For this review, take the finished solid that the model builds, in its own axes (mm). A direction names the side the tool comes from. Round coordinates to 2 decimals unless told otherwise and drop trailing zeros. Write each loop counter-clockwise with the first axis right and the second up, starting at its lowest first coordinate (ties: lowest second). Pieces come first, ordered by that corner, then holes. Notation, with made-up numbers: (-18, 36.5) - (-13, 36.5) arc R21 cw to (-13, 74.5) - close; hole circle Ø7 at (49, 31.5). An arc over 180 degrees is marked (long way). Answer in a Markdown table with one row per item. Add a question column.
from build123d import *

# Parameters (mm, degrees)
BOSS_EXTRUDE1_DEPTH             = 20
SKETCH6_R                       = 12.25
BOSS_EXTRUDE2_DEPTH             = 4.5
SKETCH4_W                       = 157.727290237
SKETCH4_H                       = 50
CUT_EXTRUDE10_DEPTH             = 34.640665044
CUT_EXTRUDE12_DEPTH             = 141.625104537
CUT_EXTRUDE12_DEPTH_BACK        = 141.625104537
SKETCH11_R                      = 10.625
SKETCH11_R_2                    = 0.95
SKETCH11_R_3                    = 0.675
CUT_EXTRUDE13_DEPTH             = 2
SKETCH12_R                      = 3.5
SKETCH12_R_2                    = 0.95
CUT_EXTRUDE14_DEPTH             = 1
CUT_EXTRUDE15_REACH             = 153.797
SKETCH14_R                      = 5
CUT_EXTRUDE16_DEPTH             = 124.889930448
CUT_EXTRUDE17_DEPTH             = 108.475579093
CUT_EXTRUDE17_DRAFT             = -2.1
CUT_EXTRUDE17_PROFILE_2_DEPTH   = 108.475579093
CUT_EXTRUDE17_PROFILE_2_DRAFT   = -2.1
CUT_EXTRUDE18_REACH             = 151.086
SKETCH16_R                      = 1
SKETCH18_R                      = 6.25
BOSS_EXTRUDE4_DEPTH             = 5.5
BOSS_EXTRUDE4_DEPTH_BACK        = 4
SKETCH19_W                      = 13
SKETCH19_H                      = 3.5
BOSS_EXTRUDE5_DEPTH             = 21.3
BOSS_EXTRUDE5_DIRECTION_2_REACH = 125.89
SKETCH20_R                      = 7.5
BOSS_EXTRUDE6_DEPTH             = 0.75
CUT_EXTRUDE19_REACH             = 153.797
SKETCH17_R                      = 3


with BuildPart() as part:
    # Sketch1 → Boss-Extrude1 (new, symmetric)
    with BuildSketch(Plane.YZ):
        Polygon((-14.772710004, -33), (35.227289996, -33), (135.227290242, -15.19542909), (135.227290242, -11.132523186), (105.227290242, -16.473894445), (105.227290242, 16.473894445), (135.227290242, 11.132523186), (135.227290242, 15.19542909), (35.227289996, 33), (-14.772710004, 33), (-14.772710004, 29), (34.917768753, 29), (34.917768753, -29), (-14.772710004, -29), align=None)
        Polygon((40.917768753, -27.923928772), (67.072529497, -23.267185861), (67.072529497, 23.267185861), (40.917768753, 27.923928772), align=None, mode=Mode.SUBTRACT)
        Polygon((73.072529497, 22.198911609), (99.227290242, 17.542168697), (99.227290242, -17.542168697), (73.072529497, -22.198911609), align=None, mode=Mode.SUBTRACT)
    extrude(amount=BOSS_EXTRUDE1_DEPTH, both=True)

    # Sketch6 → Boss-Extrude2 (add)
    with BuildSketch(Plane.XY.offset(-29)):
        Circle(SKETCH6_R)
    extrude(amount=BOSS_EXTRUDE2_DEPTH)

    # Sketch4 → Cut-Extrude10 (cut, symmetric)
    with BuildSketch(Plane(origin=(0, 0, 0), x_dir=(0, 1, 0), z_dir=(0, 0, 1))):
        with Locations((61.363645124, 0)):
            Rectangle(SKETCH4_W, SKETCH4_H)
        with BuildLine():
            Line((35.227289996, 20), (130.476978326, 15.237515595))
            ThreePointArc((130.476978326, 15.237515595), (133.850026805, 13.689879231), (135.227290242, 10.243753901))
            Line((135.227290242, 10.243753901), (135.227290242, -10.243753901))
            ThreePointArc((135.227290242, -10.243753901), (133.850026805, -13.689879231), (130.476978326, -15.237515595))
            Line((130.476978326, -15.237515595), (35.227289996, -20))
            Line((35.227289996, -20), (-2.499999995, -20))
            ThreePointArc((-2.499999995, -20), (-9.571067807, -17.071067812), (-12.499999995, -10))
            Line((-12.499999995, -10), (-12.499999995, 10))
            ThreePointArc((-12.499999995, 10), (-9.571067807, 17.071067812), (-2.499999995, 20))
            Line((-2.499999995, 20), (35.227289996, 20))
        make_face(mode=Mode.SUBTRACT)
    extrude(amount=CUT_EXTRUDE10_DEPTH, both=True, mode=Mode.SUBTRACT)

    # Sketch8 → Cut-Extrude12 (cut, two sides)
    with BuildSketch(Plane(origin=(0, 0, 0), x_dir=(0, 1, 0), z_dir=(0, 0, 1))) as cut_extrude12_sk:
        with BuildLine():
            Line((117.127290242, 4.875), (127.127290242, 4.875))
            ThreePointArc((127.127290242, 4.875), (132.002290242, 0), (127.127290242, -4.875))
            Line((127.127290242, -4.875), (117.127290242, -4.875))
            ThreePointArc((117.127290242, -4.875), (112.252290242, 0), (117.127290242, 4.875))
        make_face()
    extrude(amount=CUT_EXTRUDE12_DEPTH, mode=Mode.SUBTRACT)
    extrude(cut_extrude12_sk.sketch, amount=-CUT_EXTRUDE12_DEPTH_BACK, mode=Mode.SUBTRACT)

    # Sketch11 → Cut-Extrude13 (cut)
    with BuildSketch(Plane.XY.offset(-24.5)):
        Circle(SKETCH11_R)
        Circle(SKETCH11_R_2, mode=Mode.SUBTRACT)
        with Locations(Location((2.545584412, 7.353910524, 0), (0, 0, 180))):
            Circle(SKETCH11_R_3, mode=Mode.SUBTRACT)
        with Locations(Location((4.949747468, 4.949747468, 0), (0, 0, 180))):
            Circle(SKETCH11_R_3, mode=Mode.SUBTRACT)
        with Locations((-2.545584412, 7.353910524)):
            Circle(SKETCH11_R_3, mode=Mode.SUBTRACT)
        with Locations((-4.949747468, 4.949747468)):
            Circle(SKETCH11_R_3, mode=Mode.SUBTRACT)
        with Locations(Location((-7.353910524, 2.545584412, 0), (0, 0, 180))):
            Circle(SKETCH11_R_3, mode=Mode.SUBTRACT)
        with Locations(Location((-4.949747468, -4.949747468, 0), (0, 0, 180))):
            Circle(SKETCH11_R_3, mode=Mode.SUBTRACT)
        with Locations(Location((-2.545584412, -7.353910524, 0), (0, 0, 180))):
            Circle(SKETCH11_R_3, mode=Mode.SUBTRACT)
        with Locations(Location((7.353910524, -2.545584412, 0), (0, 0, 180))):
            Circle(SKETCH11_R_3, mode=Mode.SUBTRACT)
        with Locations((2.545584412, -7.353910524)):
            Circle(SKETCH11_R_3, mode=Mode.SUBTRACT)
        with Locations((4.949747468, -4.949747468)):
            Circle(SKETCH11_R_3, mode=Mode.SUBTRACT)
    extrude(amount=-CUT_EXTRUDE13_DEPTH, mode=Mode.SUBTRACT)

    # Sketch12 → Cut-Extrude14 (cut)
    with BuildSketch(Plane.XY.offset(-26.5)):
        Circle(SKETCH12_R)
        Circle(SKETCH12_R_2, mode=Mode.SUBTRACT)
    extrude(amount=-CUT_EXTRUDE14_DEPTH, mode=Mode.SUBTRACT)

    # Sketch13 → Cut-Extrude15 (cut, up to next)
    with BuildSketch(Plane(origin=(0, 0, -33), x_dir=(1, 0, 0), z_dir=(0, 0, -1)), mode=Mode.PRIVATE) as cut_extrude15_sk1:
        with BuildLine():
            Line((-9, 12.499999995), (-20, 12.499999995))
            Line((-20, 12.499999995), (-20, -21.500000005))
            ThreePointArc((-20, -21.500000005), (-19.160251472, -18.726499024), (-16.923076923, -16.88461539))
            ThreePointArc((-16.923076923, -16.88461539), (-13.343597645, -13.937601575), (-12, -9.500000005))
            Line((-12, -9.500000005), (-12, 9.499999995))
            ThreePointArc((-12, 9.499999995), (-11.121320344, 11.621320339), (-9, 12.499999995))
        make_face()
    cut_extrude15_tool1 = extrude(cut_extrude15_sk1.sketch, amount=-CUT_EXTRUDE15_REACH, mode=Mode.PRIVATE) & part.part
    add(cut_extrude15_tool1.solids().sort_by_distance((-16.130851, 1.777121, -33))[0], mode=Mode.SUBTRACT)

    # Sketch14 → Cut-Extrude16 (cut, through all)
    with BuildSketch(Plane(origin=(0, 105.227290242, 0), x_dir=(-1, 0, 0), z_dir=(0, 1, 0))):
        with Locations(Location((0, 0, 0), (0, 0, 90))):
            Circle(SKETCH14_R)
    extrude(amount=-CUT_EXTRUDE16_DEPTH, mode=Mode.SUBTRACT)


with BuildPart() as cut_extrude17_tool:
    # Sketch15 → Cut-Extrude17 (with draft: the straight prism first)
    with BuildSketch(Plane.XZ.offset(-34.917768753)):
        with BuildLine():
            Line((-22.502320086, 32.227030747), (-22.502320086, -32.227030747))
            ThreePointArc((-22.502320086, -32.227030747), (-10.730823709, 0), (-22.502320086, 32.227030747))
        make_face()
    extrude(amount=-CUT_EXTRUDE17_DEPTH)
    # Cut-Extrude17: the draft: its side faces are tilted about the plane it starts from
    cut_extrude17_sides = [cut_extrude17_tool.faces().sort_by_distance(p)[0] for p in [
        (-22.502320086, 89.155558299, 0),
        (-10.730823709, 89.155558299, 0),
    ]]
    draft(cut_extrude17_sides, Plane.XZ.offset(-34.917768753), CUT_EXTRUDE17_DRAFT)


with BuildPart() as part_1:
    add(part.part)

    # Cut-Extrude17: cut by cut_extrude17_tool
    add(cut_extrude17_tool.part, mode=Mode.SUBTRACT)


with BuildPart() as cut_extrude17_profile_2_tool:
    # Sketch15 → Cut-Extrude17 profile 2 (with draft: the straight prism first)
    with BuildSketch(Plane.XZ.offset(-34.917768753)):
        with BuildLine():
            ThreePointArc((22.502320086, 32.227030747), (10.730823709, 0), (22.502320086, -32.227030747))
            Line((22.502320086, -32.227030747), (22.502320086, 32.227030747))
        make_face()
    extrude(amount=-CUT_EXTRUDE17_PROFILE_2_DEPTH)
    # Cut-Extrude17 profile 2: the draft: its side faces are tilted about the plane it starts from
    cut_extrude17_profile_2_sides = [cut_extrude17_profile_2_tool.faces().sort_by_distance(p)[0] for p in [
        (22.502320086, 89.155558299, 0),
        (10.730823709, 89.155558299, 0),
    ]]
    draft(cut_extrude17_profile_2_sides, Plane.XZ.offset(-34.917768753), CUT_EXTRUDE17_PROFILE_2_DRAFT)


with BuildPart() as part_2:
    add(part_1.part)

    # Cut-Extrude17 profile 2: cut by cut_extrude17_profile_2_tool
    add(cut_extrude17_profile_2_tool.part, mode=Mode.SUBTRACT)

    # Sketch16 → Cut-Extrude18 (cut, up to next)
    with BuildSketch(Plane.XY.offset(-26.5), mode=Mode.PRIVATE) as cut_extrude18_sk1:
        with Locations((-7.353910524, -2.545584412)):
            Circle(SKETCH16_R)
    cut_extrude18_tool1 = extrude(cut_extrude18_sk1.sketch, amount=-CUT_EXTRUDE18_REACH, mode=Mode.PRIVATE) & part_2.part
    # Sketch16 → Cut-Extrude18 (cut, up to next)
    with BuildSketch(Plane.XY.offset(-26.5), mode=Mode.PRIVATE) as cut_extrude18_sk2:
        with Locations((7.353910524, 2.545584412)):
            Circle(SKETCH16_R)
    cut_extrude18_tool2 = extrude(cut_extrude18_sk2.sketch, amount=-CUT_EXTRUDE18_REACH, mode=Mode.PRIVATE) & part_2.part
    add(cut_extrude18_tool1.solids().sort_by_distance((-7.353911, -2.545584, -26.5))[0], mode=Mode.SUBTRACT)
    add(cut_extrude18_tool2.solids().sort_by_distance((7.353911, 2.545584, -26.5))[0], mode=Mode.SUBTRACT)

    # Sketch18 → Boss-Extrude4 (add, two sides)
    with BuildSketch(Plane(origin=(0, 0, 29), x_dir=(1, 0, 0), z_dir=(0, 0, -1))) as boss_extrude4_sk:
        with Locations(Location((0, 0, 0), (0, 0, 270))):
            Circle(SKETCH18_R)
    extrude(amount=BOSS_EXTRUDE4_DEPTH)
    extrude(boss_extrude4_sk.sketch, amount=-BOSS_EXTRUDE4_DEPTH_BACK)

    # Sketch19 → Boss-Extrude5 (add)
    with BuildSketch(Plane(origin=(0, 105.227290242, 0), x_dir=(-1, 0, 0), z_dir=(0, 1, 0))):
        Rectangle(SKETCH19_W, SKETCH19_H)
    extrude(amount=BOSS_EXTRUDE5_DEPTH)

    # Boss-Extrude5 direction 2: up to this face of the body (flat: up to its plane)
    boss_extrude5_direction_2_end = Plane(part_2.part.faces().sort_by_distance((0, 99.227290242, 17.061388609))[0])
    # Sketch19 → Boss-Extrude5 direction 2 (add, up to the picked face)
    with BuildSketch(Plane(origin=(0, 105.227290242, 0), x_dir=(-1, 0, 0), z_dir=(0, 1, 0)), mode=Mode.PRIVATE) as boss_extrude5_direction_2_sk1:
        Rectangle(SKETCH19_W, SKETCH19_H)
    boss_extrude5_direction_2_tool1 = split(extrude(boss_extrude5_direction_2_sk1.sketch, amount=-BOSS_EXTRUDE5_DIRECTION_2_REACH, mode=Mode.PRIVATE), bisect_by=boss_extrude5_direction_2_end, keep=Keep.BOTH, mode=Mode.PRIVATE)
    add(boss_extrude5_direction_2_tool1.solids().sort_by(Axis((0, 105.22729, 0), (0, -1, 0)))[0])

    # Sketch20 → Boss-Extrude6 (add)
    with BuildSketch(Plane(origin=(0, 0, 23.5), x_dir=(1, 0, 0), z_dir=(0, 0, -1))):
        with Locations(Location((0, 0, 0), (0, 0, 270))):
            Circle(SKETCH20_R)
    extrude(amount=-BOSS_EXTRUDE6_DEPTH)

    # Sketch17 → Cut-Extrude19 (cut, up to next)
    with BuildSketch(Plane.XY.offset(33), mode=Mode.PRIVATE) as cut_extrude19_sk1:
        with Locations((7.353910524, 2.545584412)):
            Circle(SKETCH17_R)
    cut_extrude19_tool1 = extrude(cut_extrude19_sk1.sketch, amount=-CUT_EXTRUDE19_REACH, mode=Mode.PRIVATE) & part_2.part
    # Sketch17 → Cut-Extrude19 (cut, up to next)
    with BuildSketch(Plane.XY.offset(33), mode=Mode.PRIVATE) as cut_extrude19_sk2:
        with Locations((-7.353910524, -2.545584412)):
            Circle(SKETCH17_R)
    cut_extrude19_tool2 = extrude(cut_extrude19_sk2.sketch, amount=-CUT_EXTRUDE19_REACH, mode=Mode.PRIVATE) & part_2.part
    add(cut_extrude19_tool1.solids().sort_by_distance((7.353911, 2.545584, 33))[0], mode=Mode.SUBTRACT)
    add(cut_extrude19_tool2.solids().sort_by_distance((-7.353911, -2.545584, 33))[0], mode=Mode.SUBTRACT)


solid = part_2.part
Q1. To check wall thickness, follow probe 1 along Y at (x, z) = (3, -4.5); probe 2 along Z at (x, y) = (-9, 3); probe 3 along Z at (x, y) = (4, 103). State the ranges of each line that lie inside material, in increasing order.
Q2. Add section C-C on y = 120. State the section outline as (x, z) points (3 decimals).
Q3. Insertion check: pin 1 Ø10 at (x, z) = (-11.5, -4.5) entering from -Y; pin 2 Ø4 at (y, z) = (117.5, 0.5) entering from -X; pin 3 Ø5 at (x, y) = (10.5, 80) entering from -Z. Each pin has a flat end and moves straight along its axis. Give the tip position at first contact, or say it passes through.
Q4. Draft analysis for pull direction Z (two halves, no side actions). For faces 1 (the face through (1, -12.5, -31)), 2 (the face through (0.24, 86.33, -19.84)), 3 (the face through (-11, -1, -24.5)), state which applies: released by +Z, released by -Z, zero draft, split by the parting line, or undercut.
Q5. Add section D-D on y = 102. State the section outline as (x, z) points.
Q6. Tool access review of faces 4 (the face through (2.143, -5.871, 26.658)), 5 (the face through (0.107, 112.253, 16.786)), 6 (the face through (-2.143, 5.871, 26.658)), 7 (the face through (0.27, 53.81, -25.63)), 8 (the face through (0.107, 112.253, -16.786)): name each direction out of +Z, -Z, +X, -X, +Y, -Y from which nothing blocks a thin tool from reaching the whole face with its end or side.
Q7. Add section B-B on z = 0. State the section outline as (x, y) points, then the cut area to 3 significant figures.
Q8. Add section A-A on y = 27. State the section outline as (x, z) points.
Answer sheet:
| question | item | result |
|---|---|---|
| 1 | probe 1 | y = 34.92 to 40.92, 67.07 to 73.07, 99.23 to 105.23 |
| 1 | probe 2 | z = -33 to -26.5, 29 to 33 |
| 1 | probe 3 | z = -20.93 to -3, -1.75 to 1.75, 3 to 20.93 |
| 2 | outline | (-15.761, -17.907) - (-4.875, -17.907) - (-4.875, -13.844) - (-15.761, -13.844) - close; (-15.761, 13.844) - (-4.875, 13.844) - (-4.875, 17.907) - (-15.761, 17.907) - close; (-6.5, -1.75) - (6.5, -1.75) - (6.5, 1.75) - (-6.5, 1.75) - close; (4.875, -17.907) - (15.761, -17.907) - (15.761, -13.844) - (4.875, -13.844) - close; (4.875, 13.844) - (15.761, 13.844) - (15.761, 17.907) - (4.875, 17.907) - close |
| 3 | pin 1 | stops at y = 34.92 |
| 3 | pin 2 | stops at x = -6.5 |
| 3 | pin 3 | stops at z = -25.47 |
| 4 | face 1 | zero draft |
| 4 | face 2 | undercut |
| 4 | face 3 | undercut |
| 5 | outline | (-16.66, -21.11) - (16.66, -21.11) - (16.66, -17.83) arc R47.54 cw to (16.66, 17.83) - (16.66, 21.11) - (-16.66, 21.11) - (-16.66, 17.83) arc R47.54 cw to (-16.66, -17.83) - close; hole (-4.68, -1.75) arc R5 ccw to (4.68, -1.75) - close; hole (-4.68, 1.75) - (4.68, 1.75) arc R5 ccw to start |
| 6 | face 4 | -Y |
| 6 | face 5 | +Z |
| 6 | face 6 | none |
| 6 | face 7 | +X, -X |
| 6 | face 8 | -Z |
| 7 | outline | (-13.31, 105.23) - (-13.09, 99.23) - (13.09, 99.23) - (13.31, 105.23) - (6.5, 105.23) - (6.5, 126.53) - (-6.5, 126.53) - (-6.5, 105.23) - close; (-12.13, 73.07) - (-11.91, 67.07) - (-5, 67.07) - (-5, 73.07) - close; (-10.95, 40.92) - (-10.73, 34.92) - (-5, 34.92) - (-5, 40.92) - close; (5, 34.92) - (10.73, 34.92) - (10.95, 40.92) - (5, 40.92) - close; (5, 67.07) - (11.91, 67.07) - (12.13, 73.07) - (5, 73.07) - close |
| 7 | area | 590 mm² |
| 8 | outline | (-20, -33) - (20, -33) - (20, -29) - (-20, -29) - close; (-20, 29) - (20, 29) - (20, 33) - (-20, 33) - close |
